Geometry check sheet. Reference: the model listing, model coordinates, mm. Face numbers are marked on the shaded views. A direction names the side the tool comes from. Give positions to 0.01 mm unless a question says otherwise; leave off trailing zeros. Loops run counter-clockwise (first coordinate to the right, second up) from the corner with the lowest first, then second, coordinate; pieces in that order, holes last. Notation, with made-up numbers: (25, -20) - (35, -20) arc R13 cw to (35, -10) - close; hole circle Ø4 at (48.5, 15). An arc over 180 degrees is marked (long way). Write item = value, one per line. Start each with the question number.
from build123d import *

# Parameters (mm, degrees)
SKETCH3_W = 14
SKETCH3_H = 1.980384758
SKETCH8_W = 3.9
SKETCH8_H = 5


with BuildPart() as part:
    # Sketch3 → Revolve1 (revolve)
    with BuildSketch(Plane(origin=(0, 0, 0), x_dir=(0, 0, -1), z_dir=(1, 0, 0)), mode=Mode.PRIVATE) as revolve1_sk:
        with Locations((-7, 0.990192379)):
            Rectangle(SKETCH3_W, SKETCH3_H)
    revolve(revolve1_sk.sketch.rotate(Axis((0, 0, 0), (0, 0, -1)), 90), axis=Axis((0, 0, 0), (0, 0, -1)))

    # Sketch8 → Revolve2 (revolve)
    with BuildSketch(Plane(origin=(0, 0, 0), x_dir=(0, 0, -1), z_dir=(1, 0, 0)), mode=Mode.PRIVATE) as revolve2_sk:
        with Locations((-15.95, 2.5)):
            Rectangle(SKETCH8_W, SKETCH8_H)
    revolve(revolve2_sk.sketch.rotate(Axis((0, 0, 0), (0, 0, 1)), 90), axis=Axis((0, 0, 0), (0, 0, 1)))

    # Sketch11 → Cut-Revolve3 (revolve, cut)
    with BuildSketch(Plane(origin=(0, 0, 0), x_dir=(0, 0, -1), z_dir=(1, 0, 0)), mode=Mode.PRIVATE) as cut_revolve3_sk:
        with BuildLine():
            Line((-15.632664285, 5), (-14.702, 5))
            ThreePointArc((-14.702, 5), (-14.20561104, 4.79438896), (-14, 4.298))
            Line((-14, 4.298), (-13.365, 4.298))
            Line((-13.365, 4.298), (-13.365, 5.635))
            Line((-13.365, 5.635), (-18.535, 5.635))
            Line((-18.535, 5.635), (-18.535, 0))
            Line((-18.535, 0), (-17.9, 0))
            ThreePointArc((-17.9, 0), (-17.454099823, 2.527320184), (-16.170243589, 4.749455969))
            ThreePointArc((-16.170243589, 4.749455969), (-15.929212687, 4.934288492), (-15.632664285, 5))
        make_face()
    revolve(cut_revolve3_sk.sketch.rotate(Axis((0, 0, 17.9), (0, 0, -1)), 180), axis=Axis((0, 0, 17.9), (0, 0, -1)), mode=Mode.SUBTRACT)


solid = part.part
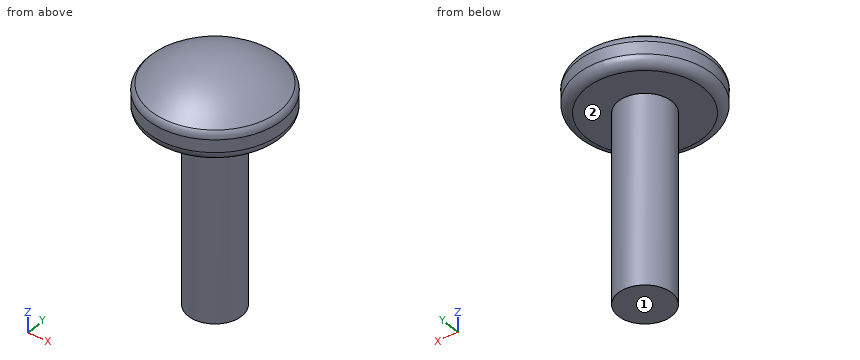
1) Tool access check on the marked faces 1 and 2. Record the directions out of +Z, -Z, +X, -X, +Y, -Y that give a thin tool (end or side, any length) a straight path to the whole face; none if there is none.
2) Material ranges on line 1 along Z through (x, y) = (1.25, -3); line 2 along Z through (x, y) = (-1, 0.5); line 3 along X through (y, z) = (0.5, 12), recorded low to high.
3) Gauge pin test, flat ends, axial feed: P1, Ø1.5, axis at x = -2.5, y = 2, coming from the -Z side; P2, Ø3, axis at y = -2.5, z = 8.5, coming from the +X side; P3, Ø2.5, axis at x = 1.5, y = 1.5, coming from the -Z side; P4, Ø3, axis at x = -2.5, y = 3.5, coming from the +Z side. Record the tip position at first contact, or that the pin passes through.
4) Cross-section at C-C on z = 5.25. Enter the section's corners in (x, y).
5) Cross-section at A-A on y = 0. Enter the section's corners in (x, z), and give its area (3 significant figures).
Checked values:
q1.face_1 = -Z, +X, -X, +Y, -Y
q1.face_2 = -Z
q2.line_1 = 14 to 17.15
q2.line_2 = 0 to 17.81
q2.line_3 = -1.92 to 1.92
q3.P1 = 14
q3.P2 = 1.71
q3.P3 = 0
q3.P4 = 17.35
q4.outline = circle Ø3.96 at (0, 0)
q5.outline = (-5, 14.7) arc R0.7 ccw to (-4.3, 14) - (-1.98, 14) - (-1.98, 0) - (1.98, 0) - (1.98, 14) - (4.3, 14) arc R0.7 ccw to (5, 14.7) - (5, 15.63) arc R0.7 ccw to (4.75, 16.17) arc R7.39 ccw to (-4.75, 16.17) arc R0.7 ccw to (-5, 15.63) - close
q5.area = 88.1 mm²
